```python
from build123d import *

# Parameters (mm, degrees)
F0_W      = 150
F0_H      = 60
F1_DEPTH  = 25
F2_W      = 146
F2_H      = 21
F3_DEPTH  = 2
F4_R      = 11.55
F5_DEPTH  = 59.1
F6_R      = 12.5
F7_DEPTH  = 6.9
F8_W      = 4
F8_H      = 8
F8_H_2    = 28.7938314093
F8_W_2    = 17.2490148246
F8_H_3    = 2.5750142522
F8_W_3    = 9
F8_H_4    = 18.5084169569
F9_DEPTH  = 35.6
F10_W     = 8
F10_H     = 28.7938314093
F10_H_2   = 18.5084169569
F10_H_3   = 8
F10_W_2   = 0.5
F10_H_4   = 15.327197553
F10_W_3   = 16.7490148246
F10_H_5   = 2.5750142522
F10_H_6   = 31.2061685907
F10_H_7   = 15.9334027047
F10_H_8   = 12.6977516338
F10_H_9   = 42.0977881948
F11_DEPTH = 2.5


with BuildPart() as f1:
    # F0 (on Front) → F1 (new body)
    with BuildSketch(Plane.XZ):
        with Locations((0, 8.6096065703)):
            Rectangle(F0_W, F0_H)
    extrude(amount=F1_DEPTH)

    # F2 (on face) → F3 (join)
    with BuildSketch(Plane.XY.offset(38.6096065703)):
        with Locations((0, -12.5)):
            Rectangle(F2_W, F2_H)
    extrude(amount=-F3_DEPTH)

    # F4 (on face) → F5 (cut)
    with BuildSketch(Plane.XY.offset(38.6096065703)):
        with Locations((60, -12.5)):
            Circle(F4_R)
        with Locations((-60, -12.5)):
            Circle(F4_R)
        with Locations((0, -12.5)):
            Circle(F4_R)
    extrude(amount=-F5_DEPTH, mode=Mode.SUBTRACT)

    # F6 (on face) → F7 (cut)
    with BuildSketch(Plane(origin=(0, 0, 0), x_dir=(-1, 0, 0), z_dir=(0, 1, 0))):
        with Locations((-58, 13.6096065703)):
            Circle(F6_R)
        with Locations((38, 13.6096065703)):
            Circle(F6_R)
    extrude(amount=-F7_DEPTH, mode=Mode.SUBTRACT)

    # F8 (on face) → F9 (cut)
    with BuildSketch(Plane.XZ.offset(25)):
        with Locations((-62, 23.4421596825)):
            Rectangle(F8_W, F8_H)
        with Locations((-58, 23.4421596825)):
            Rectangle(F8_W, F8_H)
        with Locations((-62, -6.9934777251)):
            Rectangle(F8_W, F8_H_2)
        with Locations((-58, -6.9934777251)):
            Rectangle(F8_W, F8_H_2)
        with Locations((-36.3754925877, -4.7756887507)):
            Rectangle(F8_W_2, F8_H_3)
        with Locations((-23.6245074123, 21.3886967395)):
            Rectangle(F8_W_2, F8_H_3)
        Polygon((4, 38.6096065703), (-4, 38.6096065703), (-4, 20.1011896133), (0, 20.1011896133), (4, 20.1011896133), align=None)
        with Locations((-10.5, -6.9934777251)):
            Rectangle(F8_W_3, F8_H_2)
        with Locations((10.5, -6.9934777251)):
            Rectangle(F8_W_3, F8_H_2)
        with Locations((19.5, -6.9934777251)):
            Rectangle(F8_W_3, F8_H_2)
        with Locations((32, 29.3553980918)):
            Rectangle(F8_W, F8_H_4)
        with Locations((28, 29.3553980918)):
            Rectangle(F8_W, F8_H_4)
        Polygon((36, 7.4034379795), (36, -21.3903934297), (45, -21.3903934297), (45, -6.0631958768), (45, -3.4881816246), (45, 7.4034379795), align=None)
        with Locations((53.6245074123, -4.7756887507)):
            Rectangle(F8_W_2, F8_H_3)
        with Locations((66.3754925877, 21.3886967395)):
            Rectangle(F8_W_2, F8_H_3)
    extrude(amount=-F9_DEPTH, mode=Mode.SUBTRACT)

    # F10 (on face) → F11 (cut)
    with BuildSketch(Plane.XZ.offset(25)):
        with Locations((-60, -6.9934777251)):
            Rectangle(F10_W, F10_H)
        with Locations((0, 29.3553980918)):
            Rectangle(F10_W, F10_H_2)
        with Locations((30, 29.3553980918)):
            Rectangle(F10_W, F10_H_2)
        with Locations((-60, 23.4421596825)):
            Rectangle(F10_W, F10_H_3)
        with Locations((-44.75, -13.7267946533)):
            Rectangle(F10_W_2, F10_H_4)
        with Locations((-36.1254925877, -4.7756887507)):
            Rectangle(F10_W_3, F10_H_5)
        with Locations((-23.8745074123, 21.3886967395)):
            Rectangle(F10_W_3, F10_H_5)
        Polygon((-15, 7.4034379795), (-15, -21.3903934297), (-6, -21.3903934297), (-6, 7.4034379795), (-14.5, 7.4034379795), align=None)
        Polygon((6, 7.4034379795), (6, -21.3903934297), (14.3485692441, -21.3903934297), (14.3485692441, 7.4034379795), (13.8485692441, 7.4034379795), align=None)
        Polygon((14.3485692441, 7.4034379795), (14.3485692441, -21.3903934297), (24, -21.3903934297), (24, 7.4034379795), (14.8485692441, 7.4034379795), align=None)
        with Locations((-44.75, -4.7756887507)):
            Rectangle(F10_W_2, F10_H_5)
        Polygon((36, 7.4034379795), (36, -21.3903934297), (45, -21.3903934297), (45, -6.0631958768), (45, -3.4881816246), (45, 7.4034379795), (44.5, 7.4034379795), align=None)
        with Locations((45.25, 23.0065222749)):
            Rectangle(F10_W_2, F10_H_6)
        with Locations((44.75, 23.0065222749)):
            Rectangle(F10_W_2, F10_H_6)
        with Locations((14.5985692441, 23.0065222749)):
            Rectangle(F10_W_2, F10_H_6)
        with Locations((14.0985692441, 23.0065222749)):
            Rectangle(F10_W_2, F10_H_6)
        Polygon((-14.5, 38.6096065703), (-15, 38.6096065703), (-15, 22.6762038656), (-15, 20.1011896133), (-15, 7.4034379795), (-14.5, 7.4034379795), align=None)
        with Locations((-15.25, 30.6429052179)):
            Rectangle(F10_W_2, F10_H_7)
        with Locations((-15.25, 13.7523137964)):
            Rectangle(F10_W_2, F10_H_8)
        with Locations((-15.25, 21.3886967395)):
            Rectangle(F10_W_2, F10_H_5)
        with Locations((-44.75, 17.5607124729)):
            Rectangle(F10_W_2, F10_H_9)
        Polygon((-45, 38.6096065703), (-45.5, 38.6096065703), (-45.5, -21.3903934297), (-45, -21.3903934297), (-45, -6.0631958768), (-45, -3.4881816246), align=None)
    extrude(amount=-F11_DEPTH, mode=Mode.SUBTRACT)


solid = f1.part
```
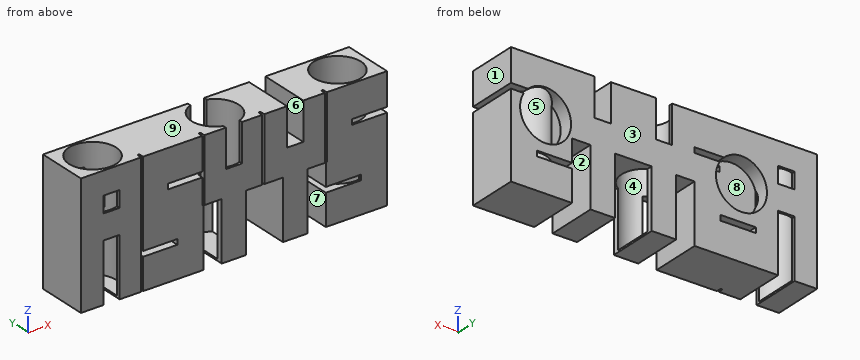
Build history of the part. All positions in model axes, mm. Face numbers are marked on the shaded views. A direction names the side the tool comes from. Give positions to 0.01 mm unless a question says otherwise; leave off trailing zeros. Order: outer loops, then holes, each group sorted by start corner. A loop starts at its lowest first (then second) coordinate and runs counter-clockwise, first axis right, second up. Notation, with made-up numbers: M 30.5,38 L 61.5,38 A14 cw 61.5,55 Z; hole C -33.5,-16 d10. An arc over 180 degrees is marked long. Write item = value, one per line. Start each with the question number.
(1) Which spindle directions (+Z, -Z, +X, -X, +Y, -Y) get a long thin tool onto all of the face, cutting with end or side? Do the marked faces 5, 6, 7, 8 and 9. Say none if no direction does.
(2) Slice it at B-B on x = -60. Write the cut outline in (y, z).
(3) Probe L1, parallel to Z at x = -38, y = -2; L2, parallel to X at y = -12, z = -1; L3, parallel to Z at x = -20, y = -9.5. List the from-to ranges inside material, lowest first. Write a range as [from, to].
(4) Slice it at A-A on z = 29.5. State how many separate pieces and enclosed holes the cut face has, plus the area to 3 significant figures.
(5) Two-plate mould, pull along X, no slides. Class the marked faces 1, 2, 3 and 4: released by +X, released by -X, zero draft, split by the parting line, or undercut.
(6) Slice it at C-C on x = -38. Write the cut outline in (y, z), plus the area to 3 significant figures.
(7) Pin check, flat tips, straight feed: pin 1 Ø1.3 at (x, y) = (1.5, -1) entering from +Z; pin 2 Ø1.8 at (y, z) = (-0.5, 22) entering from +X; pin 3 Ø5.5 at (x, y) = (16.5, -16) entering from -Z. Stop position of each tip, or through.
Responses:
q1.face_5 = +Z
q1.face_6 = +Z, +Y, -Y
q1.face_7 = -Z, +Y, -Y
q1.face_8 = +Y
q1.face_9 = +Z, +X, -X, +Y, -Y
q2.outline = M -25,7.4 L -24.05,7.4 L -24.05,19.44 L -25,19.44 Z; M -25,27.44 L -24.05,27.44 L -24.05,38.61 L -25,38.61 Z; M -0.95,7.4 L 0,7.4 L 0,19.44 L -0.95,19.44 Z; M -0.95,27.44 L 0,27.44 L 0,38.61 L -0.95,38.61 Z
q3.L1 = [-21.39, -6.06], [-3.49, 1.11], [26.11, 38.61]
q3.L2 = [-75, -71.54], [-48.46, -15], [24, 36], [45, 48.46], [71.54, 75]
q3.L3 = [-21.39, 20.1], [22.68, 38.61]
q4.separate_pieces = 3
q4.enclosed_holes = 2
q4.area = 2,260 mm2
q5.face_1 = released by +X
q5.face_2 = undercut
q5.face_3 = zero draft
q5.face_4 = undercut
q6.outline = M -25,-21.39 L 0,-21.39 L 0,-6.06 L -25,-6.06 Z; M -25,-3.49 L 0,-3.49 L 0,1.11 L -6.9,1.11 L -6.9,26.11 L 0,26.11 L 0,38.61 L -25,38.61 Z
q6.area = 1,260 mm2
q7.pin_1 = 20.1
q7.pin_2 = 75
q7.pin_3 = 7.4
